Geometry check sheet. Reference: drawing and pictorial views, mm from the part's lowest x, y, z. Give positions to 0.01 mm unless a question says otherwise; leave off trailing zeros. Loops run counter-clockwise (first coordinate to the right, second up) from the corner with the lowest first, then second, coordinate; pieces in that order, holes last. Notation, with made-up numbers: (-35.5, -26.5) -> (2.5, -26.5) arc R24 ccw to (2.5, -4.5) -> close; hole circle Ø1 at (87.25, 22.25). An arc over 180 degrees is marked (long way). Write item = value, one per line. Start each with the question number.
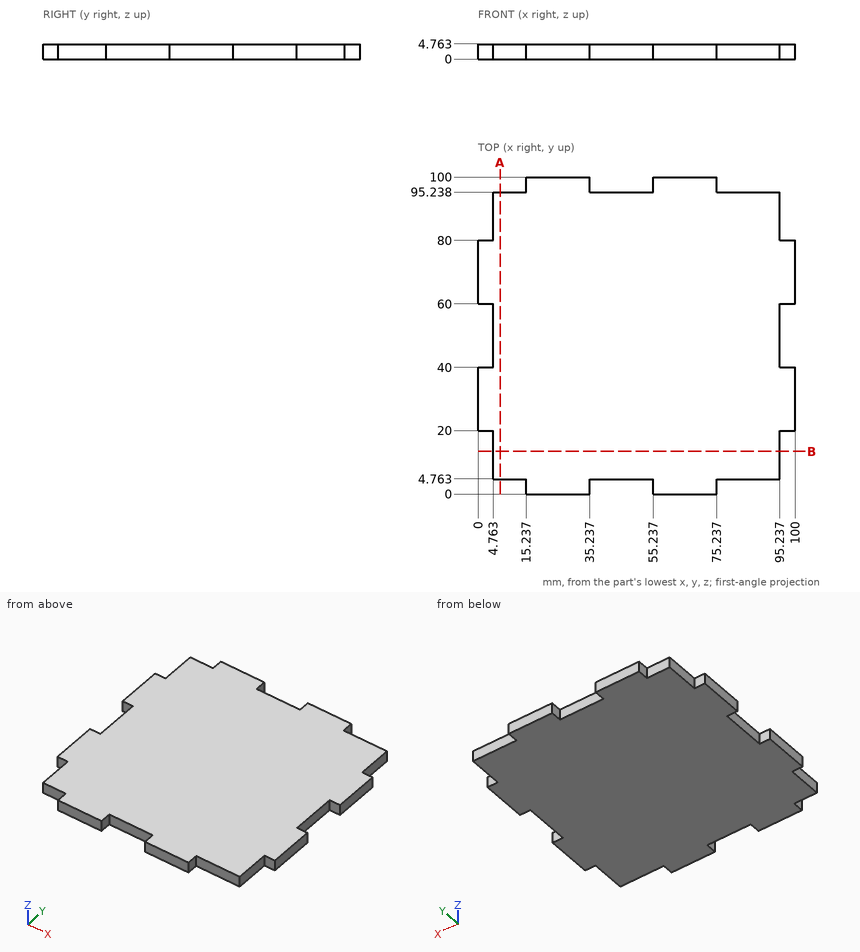
1) Depth check by flat-ended pin: pin 1 Ø1.4 at (y, z) = (2, 2) entering from -X; pin 2 Ø1.4 at (x, z) = (97, 2.5) entering from -Y; pin 3 Ø1.4 at (y, z) = (90.5, 1.5) entering from -X; pin 4 Ø1 at (y, z) = (27.5, 2.5) entering from -X. Enter the tip coordinate at first touch or a pass-through.
2) Thickness scan on line 1 (X direction, y = 88, z = 4.4). Record the ranges inside material, lowest first.
3) Section check A-A (x = 7). Enter the section's corners in (y, z).
Check result:
q1.pin_1 = 15.24
q1.pin_2 = 20
q1.pin_3 = 4.76
q1.pin_4 = 0
q2.line_1 = 4.76 to 95.24
q3.outline = (4.76, 0) -> (95.24, 0) -> (95.24, 4.76) -> (4.76, 4.76) -> close
